```python
from build123d import *

# Parameters (mm, degrees)
F0_R     = 4.445
F1_DEPTH = 3.81


with BuildPart() as f1:
    # F0 (on Top) → F1 (new body)
    with BuildSketch(Plane.XY):
        with BuildLine():
            Line((63.5, -69.652364), (-63.5, -69.652364))
            add(Edge.make_bspline(
                [(-63.5, -69.652364), (-27.377963, -103.611864), (29.017352, -104.595505), (63.5, -69.652364)],
                knots=[0, 0, 0, 0, 127, 127, 127, 127], degree=3))
        make_face()
        with BuildLine():
            add(Edge.make_bspline(
                [(0, 40.332863), (49.345907, 25.572751), (76.559924, -21.641931), (63.5, -69.652364)],
                knots=[0, 0, 0, 0, 127, 127, 127, 127], degree=3))
            Line((0, 40.332863), (63.5, -69.652364))
        make_face()
        Polygon((63.5, -69.652364), (0, 40.332863), (-63.5, -69.652364), align=None)
        with Locations((-50.8, -64.572364)):
            Circle(F0_R, mode=Mode.SUBTRACT)
        with Locations((50.8, -64.572364)):
            Circle(F0_R, mode=Mode.SUBTRACT)
        with BuildLine():
            Line((-19.703986, -18.950023), (-19.703986, -42.462528))
            ThreePointArc((-19.703986, -42.462528), (-23.513986, -46.272528), (-27.323986, -42.462528))
            Line((-27.323986, -42.462528), (-27.323986, -18.950023))
            ThreePointArc((-27.323986, -18.950023), (-23.513986, -15.140023), (-19.703986, -18.950023))
        make_face(mode=Mode.SUBTRACT)
        with BuildLine():
            ThreePointArc((-12.7, -19.413278), (0, -6.713278), (12.7, -19.413278))
            Line((12.7, -19.413278), (12.7, -42.692736))
            ThreePointArc((12.7, -42.692736), (0, -55.392736), (-12.7, -42.692736))
            Line((-12.7, -42.692736), (-12.7, -19.413278))
        make_face(mode=Mode.SUBTRACT)
        with BuildLine():
            Line((19.703986, -42.462528), (19.703986, -18.950023))
            ThreePointArc((19.703986, -18.950023), (23.513986, -15.140023), (27.323986, -18.950023))
            Line((27.323986, -18.950023), (27.323986, -42.462528))
            ThreePointArc((27.323986, -42.462528), (23.513986, -46.272528), (19.703986, -42.462528))
        make_face(mode=Mode.SUBTRACT)
        with Locations((0, 26.362863)):
            Circle(F0_R, mode=Mode.SUBTRACT)
        with BuildLine():
            Line((-63.5, -69.652364), (0, 40.332863))
            add(Edge.make_bspline(
                [(0, 40.332863), (-49.345907, 25.572751), (-76.559924, -21.641931), (-63.5, -69.652364)],
                knots=[0, 0, 0, 0, 127, 127, 127, 127], degree=3))
        make_face()
    extrude(amount=F1_DEPTH)


solid = f1.part
```
Geometry check sheet. Reference: the model listing, model coordinates, mm. A direction names the side the tool comes from. Coordinates: 2 decimals unless noted, no trailing zeros. One line per item, written item: value. Start each with the question number.
(1) Depth check by flat-ended pin: pin 1 (1.1 mm diameter, centred on y = -34, z = 1, fed in from -X); pin 2 (8 mm diameter, centred on x = 0, y = 26.36, fed in from +Z); pin 3 (1.9 mm diameter, centred on y = -33.5, z = 1, fed in from +X); pin 4 (1.1 mm diameter, centred on y = -32, z = 1.5, fed in from -X). Enter the tip coordinate at first touch or a pass-through.
(2) Scan lines: line 1 along Y through (x, z) = (0, 1.45); line 2 along X through (y, z) = (-32.5, 1.05); line 3 along X through (y, z) = (-39.5, 0.9). Record each from-to range of solid material in increasing order. Write a range as [from, to].
(3) Tool access check on faces 3 (the face through (16, -31, 3.81)), 4 (the face through (0.28, -55.39, 1.88)). Record the directions out of +Z, -Z, +X, -X, +Y, -Y that give a thin tool (end or side, any length) a straight path to the whole face; none if there is none.
(4) Release check for a two-part mould opening along Y. For faces 1 (the face through (55.04, -63.24, 1.88)), 2 (the face through (16, -31, 0)) record: released by +Y, released by -Y, zero draft, split by the parting line, or undercut.
(5) Sectioned sample at A-A, the plane z = 0.7. State how many separate pieces and enclosed holes the cut face has, and give its area (3 significant figures).
Filled sheet:
1. pin 1: x = -66.06
1. pin 2: through
1. pin 3: x = 66.05
1. pin 4: x = -65.78
2. line 1: [-95.49, -55.39], [-6.71, 21.92], [30.81, 40.33]
2. line 2: [-65.78, -27.32], [-19.7, -12.7], [12.7, 19.7], [27.32, 65.78]
2. line 3: [-66.55, -27.32], [-19.7, -12.7], [12.7, 19.7], [27.32, 66.55]
3. face 3: +Z, +X, -X, +Y, -Y
3. face 4: +Z, -Z
4. face 1: undercut
4. face 2: zero draft
5. separate pieces: 1
5. enclosed holes: 6
5. area: 12,100 mm²
